Verification items for the finished model (mm, model axes). A direction names the side the tool comes from. Coordinates: 2 decimals unless noted, no trailing zeros. Loops run counter-clockwise (first coordinate to the right, second up) from the corner with the lowest first, then second, coordinate; pieces in that order, holes last. Notation, with made-up numbers: (19.5, 57.25) -> (36.5, 57.25) arc R31 ccw to (36.5, 94.25) -> close; hole circle Ø7 at (6.25, -9.75). An arc over 180 degrees is marked (long way). Answer as a JSON object with one key per item and string values. Group by question number.
Q1. Gauge pin test, flat ends, axial feed: pin 1 Ø3.5 at (x, z) = (9, 17.5) entering from +Y; pin 2 Ø8 at (y, z) = (3, 10.5) entering from -X; pin 3 Ø3 at (x, z) = (1.5, 22) entering from +Y; pin 4 Ø4.5 at (x, z) = (9.5, 16.5) entering from +Y. Record the tip position at first contact, or that the pin passes through.
Q2. Cross-section at A-A on z = 17.5. Record the boundary of the cut face in (x, y), and give its area (3 significant figures).
Q3. Cross-section at D-D on z = 32.5. Record the boundary of the cut face in (x, y), and give its area (3 significant figures).
Q4. Set-up check for faces 4 (the flat face through (5, 4, 17)), 5 (the flat face through (10.43, 3.014, 20.023)), 6 (the flat face through (15, 2, 17)): record each of +Z, -Z, +X, -X, +Y, -Y from which the full face is reachable in a straight line by a thin tool's end or side.
Q5. Cross-section at C-C on x = 9.75. Record the boundary of the cut face in (y, z), and give its area (3 significant figures).
Q6. Release check for a two-part mould opening along X. For faces 1 (the flat face through (0, 8, 17)), 2 (the flat face through (2, 2, 35)), 3 (the flat face through (10.47, 3.01, 15)) record: released by +X, released by -X, zero draft, split by the parting line, or undercut.
Q7. Scan lines: L1, parallel to X at y = 1.2, z = 17.5; L2, parallel to Y at x = 11, z = 6; L3, parallel to X at y = 7.5, z = 20.5. Record each from-to range of solid material in increasing order.
Q8. Cross-section at B-B on y = 2.5. Record the boundary of the cut face in (x, z), and give its area (3 significant figures).
```python
from build123d import *

# Parameters (mm, degrees)
SALIENTE_EXTRUIR1_DEPTH = 35
CORTAR_EXTRUIR1_DEPTH   = 2
CROQUIS4_R              = 1.5
CORTAR_EXTRUIR2_DEPTH   = 10
CORTAR_EXTRUIR3_DEPTH   = 10
CORTAR_EXTRUIR4_DEPTH   = 10


with BuildPart() as part:
    # Croquis2 → Saliente-Extruir1 (new body)
    with BuildSketch(Plane.XY):
        Polygon((0, 23), (3, 23), (3, 4), (15, 4), (15, 0), (0, 0), align=None)
    extrude(amount=SALIENTE_EXTRUIR1_DEPTH)

    # Croquis3 → Cortar-Extruir1 (cut)
    with BuildSketch(Plane(origin=(0, 4, 0), x_dir=(1, 0, 0), z_dir=(0, 1, 0))):
        Polygon((9, -14.151368439), (6.1, -15.825684219), (6.1, -19.174315781), (9, -20.848631561), (11.9, -19.174315781), (11.9, -15.825684219), align=None)
    extrude(amount=-CORTAR_EXTRUIR1_DEPTH, mode=Mode.SUBTRACT)

    # Croquis4 → Cortar-Extruir2 (cut)
    with BuildSketch(Plane(origin=(0, 2, 0), x_dir=(1, 0, 0), z_dir=(0, 1, 0))):
        with Locations(Location((9, -17.5, 0), (0, 0, 270))):
            Circle(CROQUIS4_R)
    extrude(amount=-CORTAR_EXTRUIR2_DEPTH, mode=Mode.SUBTRACT)

    # Croquis5 → Cortar-Extruir3 (cut)
    with BuildSketch(Plane(origin=(0, 4, 0), x_dir=(1, 0, 0), z_dir=(0, 1, 0))):
        with BuildLine():
            Line((15, -12), (15, -23))
            ThreePointArc((15, -23), (11.485281374, -31.485281374), (3, -35))
            Line((3, -35), (3, -39.861701289))
            Line((3, -39.861701289), (21.688312252, -36.848700447))
            Line((21.688312252, -36.848700447), (27.206798155, -6.851825545))
            Line((27.206798155, -6.851825545), (15.87267332, 7.755192399))
            Line((15.87267332, 7.755192399), (3, 0))
            ThreePointArc((3, 0), (11.485281374, -3.514718626), (15, -12))
        make_face()
    extrude(amount=-CORTAR_EXTRUIR3_DEPTH, mode=Mode.SUBTRACT)

    # Croquis6 → Cortar-Extruir4 (cut)
    with BuildSketch(Plane(origin=(3, 0, 0), x_dir=(0, 0, -1), z_dir=(1, 0, 0))):
        with BuildLine():
            Line((-35, 4), (-43.463242579, 10.305944429))
            Line((-43.463242579, 10.305944429), (-37.648578304, 30.185339472))
            Line((-37.648578304, 30.185339472), (-37.331119495, 31.270679702))
            Line((-37.331119495, 31.270679702), (8.796856155, 26.447825939))
            Line((8.796856155, 26.447825939), (6.381141064, 12.03440645))
            Line((6.381141064, 12.03440645), (0, 4))
            ThreePointArc((0, 4), (-17.5, 21.5), (-35, 4))
        make_face()
    extrude(amount=-CORTAR_EXTRUIR4_DEPTH, mode=Mode.SUBTRACT)


solid = part.part
```
Computed values:
{
 "1": {"pin 1": "stops at y = 2", "pin 2": "stops at x = 0", "pin 3": "stops at y = 21.24", "pin 4": "stops at y = 4"},
 "2": {"outline": "(0, 0) -> (7.5, 0) -> (7.5, 2) -> (6.1, 2) -> (6.1, 4) -> (3, 4) -> (3, 21.5) -> (0, 21.5) -> close; (10.5, 0) -> (15, 0) -> (15, 4) -> (11.9, 4) -> (11.9, 2) -> (10.5, 2) -> close", "area": "94.9 mm²"},
 "3": {"outline": "(0, 0) -> (10.33, 0) -> (10.33, 4) -> (3, 4) -> (3, 13.01) -> (0, 13.01) -> close", "area": "68.4 mm²"},
 "4": {"face 4": "+Z, -Z, +X, +Y", "face 5": "+Y", "face 6": "+Z, -Z, +X, +Y, -Y"},
 "5": {"outline": "(0, 2.08) -> (4, 2.08) -> (4, 14.58) -> (2, 14.58) -> (2, 16.2) -> (0, 16.2) -> close; (0, 18.8) -> (2, 18.8) -> (2, 20.42) -> (4, 20.42) -> (4, 32.92) -> (0, 32.92) -> close", "area": "107 mm²"},
 "6": {"face 1": "released by -X", "face 2": "zero draft", "face 3": "undercut"},
 "7": {"L1": "x = 0 to 7.5, 10.5 to 15", "L2": "y = 0 to 4", "L3": "x = 0 to 3"},
 "8": {"outline": "(0, 0) -> (3, 0) arc R12 ccw to (15, 12) -> (15, 23) arc R12 ccw to (3, 35) -> (0, 35) -> close; hole (6.1, 15.83) -> (9, 14.15) -> (11.9, 15.83) -> (11.9, 19.17) -> (9, 20.85) -> (6.1, 19.17) -> close", "area": "434 mm²"}
}
